Build history of the part. All positions in model axes, mm. A direction names the side the tool comes from. Coordinates: 2 decimals unless noted, no trailing zeros. Order: outer loops, then holes, each group sorted by start corner. A loop starts at its lowest first (then second) coordinate and runs counter-clockwise, first axis right, second up. Notation, with made-up numbers: M -39,19.5 L -2,19.5 A5 ccw -2,27.5 Z; hole C 56,82.25 d6. An arc over 180 degrees is marked long. Write item = value, one per line. Start each with the question number.
Q1. Pull direction Z, two halves, no side cores. Call faces 1 (the face through (-3, -60, -174)), 2 (the face through (528, -30, -800)), 3 (the face through (311, -30, -280)): released by +Z, released by -Z, zero draft, split by the parting line, or undercut.
Q2. Band-saw the part on A-A on z = -365. Write the cut outline in (x, y).
Q3. 3-axis set-ups, long thin cutter, end or side, ignore diameter. For faces 4 (the face through (30, -30, 537)), 5 (the face through (-660, -20, -11)), 6 (the face through (400, -24, -770)): which of +Z, -Z, +X, -X, +Y, -Y reach the whole face in a straight line?
Q4. Drill centre lines: probe 1 along Z at (x, y) = (-577.5, -48); probe 2 along X at (y, z) = (-46.5, -391); probe 3 along Z at (x, y) = (364, -44). Where is each one in solid material? Low to high.
Q5. Band-saw the part on B-B on x = -181. Write the cut outline in (y, z).
Q6. Pin check, flat tips, straight feed: P1, Ø18, axis at x = 336.5, y = -41, coming from the -Z side; P2, Ø9.5, axis at y = -54, z = -314, coming from the -X side. Stop position of each tip, or through.
Q7. Band-saw the part on C-C on y = -50. State how many separate pieces and enclosed holes the cut face has, plus the area to 3 significant figures.
```python
from build123d import *

# Parameters (mm, degrees)
F0_W      = 1320
F0_H      = 1600
F0_W_2    = 570
F0_H_2    = 400
F0_H_3    = 560
F1_DEPTH  = 60
F2_W      = 12
F2_H      = 1600
F3_DEPTH  = 19
F5_DEPTH  = 60
F6_W      = 100
F6_H      = 60
F7_DEPTH  = 30
F8_W      = 100
F8_H      = 20
F9_DEPTH  = 30
F10_W     = 100
F10_H     = 20
F11_DEPTH = 30


with BuildPart() as f1:
    # F0 (on Front) → F1 (new body)
    with BuildSketch(Plane.XZ):
        Rectangle(F0_W, F0_H)
        with Locations((-315, -540)):
            Rectangle(F0_W_2, F0_H_2, mode=Mode.SUBTRACT)
        with Locations((315, -540)):
            Rectangle(F0_W_2, F0_H_2, mode=Mode.SUBTRACT)
        with Locations((-315, 0)):
            Rectangle(F0_W_2, F0_H_3, mode=Mode.SUBTRACT)
        with Locations((-315, 540)):
            Rectangle(F0_W_2, F0_H_2, mode=Mode.SUBTRACT)
        with Locations((315, 0)):
            Rectangle(F0_W_2, F0_H_3, mode=Mode.SUBTRACT)
        with Locations((315, 540)):
            Rectangle(F0_W_2, F0_H_2, mode=Mode.SUBTRACT)
    extrude(amount=F1_DEPTH)

    # F2 (on face) → F3 (cut)
    with BuildSketch(Plane.XZ.offset(60)):
        with Locations((-654, 0)):
            Rectangle(F2_W, F2_H)
        with Locations((654, 0)):
            Rectangle(F2_W, F2_H)
    extrude(amount=-F3_DEPTH, mode=Mode.SUBTRACT)

    # F4 (on face) → F5 (cut)
    with BuildSketch(Plane.XZ.offset(60)):
        with BuildLine():
            Line((-400, -790), (-400, -800))
            Line((-400, -800), (-300, -800))
            Line((-300, -800), (-300, -790))
            ThreePointArc((-300, -790), (-302.928932, -782.928932), (-310, -780))
            Line((-310, -780), (-390, -780))
            ThreePointArc((-390, -780), (-397.071068, -782.928932), (-400, -790))
        make_face()
        with BuildLine():
            Line((300, -790), (300, -800))
            Line((300, -800), (400, -800))
            Line((400, -800), (400, -790))
            ThreePointArc((400, -790), (397.071068, -782.928932), (390, -780))
            Line((390, -780), (310, -780))
            ThreePointArc((310, -780), (302.928932, -782.928932), (300, -790))
        make_face()
    extrude(amount=-F5_DEPTH, mode=Mode.SUBTRACT)

    # F6 (on face) → F7 (cut)
    with BuildSketch(Plane(origin=(0, 0, 0), x_dir=(-1, 0, 0), z_dir=(0, 1, 0))):
        with Locations((-350, -770)):
            Rectangle(F6_W, F6_H)
        with Locations((350, -770)):
            Rectangle(F6_W, F6_H)
    extrude(amount=-F7_DEPTH, mode=Mode.SUBTRACT)

    # F8 (on face) → F9 (cut)
    with BuildSketch(Plane(origin=(0, -30, 0), x_dir=(-1, 0, 0), z_dir=(0, 1, 0))):
        with Locations((-350, -750)):
            Rectangle(F8_W, F8_H)
    extrude(amount=-F9_DEPTH, mode=Mode.SUBTRACT)

    # F10 (on face) → F11 (cut)
    with BuildSketch(Plane(origin=(0, -30, 0), x_dir=(-1, 0, 0), z_dir=(0, 1, 0))):
        with Locations((350, -750)):
            Rectangle(F10_W, F10_H)
    extrude(amount=-F11_DEPTH, mode=Mode.SUBTRACT)


solid = f1.part
```
Recorded:
q1.face_1 = zero draft
q1.face_2 = released by -Z
q1.face_3 = undercut
q2.outline = M -660,-41 L -648,-41 L -648,-60 L -600,-60 L -600,0 L -660,0 Z; M -30,-60 L 30,-60 L 30,0 L -30,0 Z; M 600,-60 L 648,-60 L 648,-41 L 660,-41 L 660,0 L 600,0 Z
q3.face_4 = +Y, -Y
q3.face_5 = +Z, -Z, -X, +Y, -Y
q3.face_6 = +Y
q4.probe_1 = -800 to -740, -340 to -280, 280 to 340, 740 to 800
q4.probe_2 = -648 to -600, -30 to 30, 600 to 648
q4.probe_3 = -780 to -760, -340 to -280, 280 to 340, 740 to 800
q5.outline = M -60,-800 L 0,-800 L 0,-740 L -60,-740 Z; M -60,-340 L 0,-340 L 0,-280 L -60,-280 Z; M -60,280 L 0,280 L 0,340 L -60,340 Z; M -60,740 L 0,740 L 0,800 L -60,800 Z
q6.P1 = -780
q6.P2 = -648
q7.separate_pieces = 1
q7.enclosed_holes = 6
q7.area = 515,000 mm2
